```python
from build123d import *

# Parameters (mm, degrees)
SKETCH1_W           = 60
SKETCH1_H           = 31
BOSS_EXTRUDE1_DEPTH = 16
SKETCH2_W           = 16
SKETCH2_H           = 8
BOSS_EXTRUDE2_DEPTH = 5


with BuildPart() as part:
    # Sketch1 → Boss-Extrude1 (new body)
    with BuildSketch(Plane.XY):
        with Locations((30, 15.5)):
            Rectangle(SKETCH1_W, SKETCH1_H)
    extrude(amount=BOSS_EXTRUDE1_DEPTH)

    # Sketch2 → Boss-Extrude2 (add)
    with BuildSketch(Plane.ZY):
        with Locations((8, 27)):
            Rectangle(SKETCH2_W, SKETCH2_H)
    extrude(amount=BOSS_EXTRUDE2_DEPTH)


solid = part.part
```
Could you check a few things on this model? Use its own coordinates, in mm. A direction names the side the tool comes from. Give positions to 0.01 mm unless a question says otherwise; leave off trailing zeros. Order: outer loops, then holes, each group sorted by start corner. A loop starts at its lowest first (then second) coordinate and runs counter-clockwise, first axis right, second up.
Q1. I'm going to push a flat-ended pin straight in: P1, Ø2.5, axis at x = -2, z = 11, coming from the -Y side. Where does the tip first touch, or does it pass through?
Q2. Suppose I cut it at C-C, the plane y = 5. Write out the boundary of the cut face in (x, z), and give its area (3 significant figures).
Q3. Suppose I cut it at A-A, the plane z = 4. Write out the boundary of the cut face in (x, y), and give its area (3 significant figures).
Q4. For faces 1 (the flat face through (-2, 23, 8)), 2 (the flat face through (30, 0, 8)), which set-ups out of +Z, -Z, +X, -X, +Y, -Y let a thin tool reach every point of the face, with its end or its side?
Q5. Suppose I cut it at B-B, the plane x = -1. Write out the boundary of the cut face in (y, z).
Q6. If I drill on line 1 along X through (y, z) = (16, 9); line 2 along Y through (x, z) = (-1.5, 8.5), over which ranges is the centre line in solid material (lowest first)?
Solution:
1. P1: stops at y = 23
2. outline: (0, 0) - (60, 0) - (60, 16) - (0, 16) - close
2. area: 960 mm2
3. outline: (-5, 23) - (0, 23) - (0, 0) - (60, 0) - (60, 31) - (-5, 31) - close
3. area: 1,900 mm2
4. face 1: +Z, -Z, -X, -Y
4. face 2: +Z, -Z, +X, -X, -Y
5. outline: (23, 0) - (31, 0) - (31, 16) - (23, 16) - close
6. line 1: x = 0 to 60
6. line 2: y = 23 to 31
